from build123d import *

# Parameters (mm, degrees)
CROQUIS3_W                 = 106
CROQUIS3_H                 = 179
SALIENTE_EXTRUIR4_DEPTH    = 3
CROQUIS3_6_W               = 99.5
CROQUIS3_6_H               = 172.5
CROQUIS3_6_W_2             = 96.25
CROQUIS3_6_H_2             = 169.25
SALIENTE_EXTRUIR5_DEPTH    = 7
CROQUIS7_R                 = 10
CORTAR_EXTRUIR1_DEPTH      = 7
REDONDEO1_R                = 3
CORTAR_EXTRUIR2_DEPTH      = 20
CORTAR_EXTRUIR2_DEPTH_BACK = 20
CROQUIS8_R                 = 1.5
CROQUIS12_R                = 3
CORTAR_EXTRUIR3_DEPTH      = 2
CROQUIS13_R                = 2.5
SALIENTE_EXTRUIR7_DEPTH    = 1
CORTAR_EXTRUIR4_DEPTH      = 1
CORTAR_EXTRUIR4_DEPTH_BACK = 11
CROQUIS14_R                = 1.5


with BuildPart() as part:
    # Croquis3 → Saliente-Extruir4 (new body)
    with BuildSketch(Plane(origin=(0, 0, 0), x_dir=(1, 0, 0), z_dir=(0, 1, 0))):
        Rectangle(CROQUIS3_W, CROQUIS3_H)
    extrude(amount=SALIENTE_EXTRUIR4_DEPTH)

    # Croquis3_6 → Saliente-Extruir5 (add)
    with BuildSketch(Plane(origin=(0, 0, 0), x_dir=(1, 0, 0), z_dir=(0, 1, 0))):
        Rectangle(CROQUIS3_6_W, CROQUIS3_6_H)
        Rectangle(CROQUIS3_6_W_2, CROQUIS3_6_H_2, mode=Mode.SUBTRACT)
    extrude(amount=SALIENTE_EXTRUIR5_DEPTH)

    # Croquis7 → Cortar-Extruir1 (cut)
    with BuildSketch(Plane.XZ):
        with Locations(Location((28, -44.5, 0), (0, 0, 270))):
            Circle(CROQUIS7_R)
    extrude(amount=-CORTAR_EXTRUIR1_DEPTH, mode=Mode.SUBTRACT)

    # Redondeo1
    redondeo1_edges = [part.edges().sort_by_distance(p)[0] for p in [
        (53, 1.5, 89.5),
        (-53, 1.5, 89.5),
        (-53, 1.5, -89.5),
        (53, 1.5, -89.5),
    ]]
    fillet(redondeo1_edges, radius=REDONDEO1_R)

    # Croquis8 → Cortar-Extruir2 (cut, two sides: drawn at the far end of the back side and taken through both)
    with BuildSketch(Plane(origin=(0, 3, 0), x_dir=(1, 0, 0), z_dir=(0, 1, 0)).offset(-CORTAR_EXTRUIR2_DEPTH_BACK)):
        with Locations(Location((-34, 71, 0), (0, 0, 270))):
            Circle(CROQUIS8_R)
        with Locations(Location((34, 71, 0), (0, 0, 270))):
            Circle(CROQUIS8_R)
        with Locations(Location((-34, -70, 0), (0, 0, 270))):
            Circle(CROQUIS8_R)
        with Locations(Location((34, -70, 0), (0, 0, 270))):
            Circle(CROQUIS8_R)
    extrude(amount=CORTAR_EXTRUIR2_DEPTH + CORTAR_EXTRUIR2_DEPTH_BACK, mode=Mode.SUBTRACT)

    # Croquis12 → Cortar-Extruir3 (cut)
    with BuildSketch(Plane.XZ):
        with Locations(Location((-34, 70, 0), (0, 0, 270))):
            Circle(CROQUIS12_R)
        with Locations(Location((34, 70, 0), (0, 0, 270))):
            Circle(CROQUIS12_R)
        with Locations(Location((34, -71, 0), (0, 0, 270))):
            Circle(CROQUIS12_R)
        with Locations(Location((-34, -71, 0), (0, 0, 270))):
            Circle(CROQUIS12_R)
    extrude(amount=-CORTAR_EXTRUIR3_DEPTH, mode=Mode.SUBTRACT)

    # Croquis13 → Saliente-Extruir7 (add)
    with BuildSketch(Plane(origin=(0, 3, 0), x_dir=(1, 0, 0), z_dir=(0, 1, 0))):
        with Locations(Location((-34, 71, 0), (0, 0, 270))):
            Circle(CROQUIS13_R)
        with Locations(Location((34, 71, 0), (0, 0, 270))):
            Circle(CROQUIS13_R)
        with Locations(Location((-34, -70, 0), (0, 0, 270))):
            Circle(CROQUIS13_R)
        with Locations(Location((34, -70, 0), (0, 0, 270))):
            Circle(CROQUIS13_R)
    extrude(amount=SALIENTE_EXTRUIR7_DEPTH)

    # Croquis14 → Cortar-Extruir4 (cut, two sides: drawn at the far end of the back side and taken through both)
    with BuildSketch(Plane.XZ.offset(-CORTAR_EXTRUIR4_DEPTH_BACK)):
        with Locations(Location((-34, 70, 0), (0, 0, 270))):
            Circle(CROQUIS14_R)
        with Locations(Location((34, 70, 0), (0, 0, 270))):
            Circle(CROQUIS14_R)
        with Locations(Location((34, -71, 0), (0, 0, 270))):
            Circle(CROQUIS14_R)
        with Locations(Location((-34, -71, 0), (0, 0, 270))):
            Circle(CROQUIS14_R)
    extrude(amount=CORTAR_EXTRUIR4_DEPTH + CORTAR_EXTRUIR4_DEPTH_BACK, mode=Mode.SUBTRACT)


solid = part.part
Could you check a few things on this model? Use its own coordinates, in mm. A direction names the side the tool comes from. Give positions to 0.01 mm unless a question says otherwise; leave off trailing zeros. Order: outer loops, then holes, each group sorted by start corner. A loop starts at its lowest first (then second) coordinate and runs counter-clockwise, first axis right, second up. Notation, with made-up numbers: M -38.5,38 L 12.5,38 A12 cw 12.5,61 Z; hole C 89.5,39 d8. An arc over 180 degrees is marked long. One line per question, with ' | ' between items.
1. We'd pull the mould along X, two halves only. Please class faces 1 (the face through (-1, 0, -1)), 2 (the face through (-31.97, 0.99, 72.21)), 3 (the face through (-49.75, 5, 1)), 4 (the face through (35.69, 3.49, 68.16)): +X half, -X half, draft (parallel to the pull), parting line (faces both ways), or undercut.
Results:
face 1: draft | face 2: undercut | face 3: -X half | face 4: undercut
2. I want a section at C-C (z = -18.5). List the corners of the cut face in (x, y) for me (3 decimals).
Results:
outline: M -53,0 L 53,0 L 53,3 L 49.75,3 L 49.75,7 L 48.125,7 L 48.125,3 L -48.125,3 L -48.125,7 L -49.75,7 L -49.75,3 L -53,3 Z
3. I want a section at A-A (z = -44.5). List the corners of the cut face in (x, y) for me (3 decimals), and give its area (3 significant figures).
Results:
outline: M -53,0 L 18,0 L 18,3 L -48.125,3 L -48.125,7 L -49.75,7 L -49.75,3 L -53,3 Z; M 38,0 L 53,0 L 53,3 L 49.75,3 L 49.75,7 L 48.125,7 L 48.125,3 L 38,3 Z | area: 271 mm²
4. If I drill on line 1 (X direction, y = 0.5, z = 70); line 2 (Z direction, x = -37, y = 5) (3 decimals); line 3 (X direction, y = 4.5, z = 17.5) (3 decimals), over which ranges is the centre line in solid material (lowest first)?
Results:
line 1: -53 to -37, -31 to 31, 37 to 53 | line 2: -86.25 to -84.625, 84.625 to 86.25 | line 3: -49.75 to -48.125, 48.125 to 49.75
5. I want a section at B-B (x = -22). List the corners of the cut face in (y, z) for me (3 decimals), and give its area (3 significant figures).
Results:
outline: M 0,-89.5 L 3,-89.5 L 3,-86.25 L 7,-86.25 L 7,-84.625 L 3,-84.625 L 3,84.625 L 7,84.625 L 7,86.25 L 3,86.25 L 3,89.5 L 0,89.5 Z | area: 550 mm²
6. I'm going to push flat-ended pins straight in: pin 1 (1.2 mm diameter, centred on y = 5.5, z = -29.5, fed in from -X); pin 2 (1.2 mm diameter, centred on y = 4, z = -42.5, fed in from +X); pin 3 (5 mm diameter, centred on x = -11.5, z = 37.5, fed in from +Y); pin 4 (1.5 mm diameter, centred on x = 34, z = -71.5, fed in from +Y) (1 decimal). Where does each tip first touch, or does it pass through?
Results:
pin 1: x = -49.75 | pin 2: x = 49.75 | pin 3: y = 3 | pin 4: through
7. For faces 5 (the face through (-1, 5, 86.25)), 6 (the face through (32.7, 2, 68.7)), 7 (the face through (-34, 4, -69)), 8 (the face through (21.92, 1.48, -36.56)), which set-ups out of +Z, -Z, +X, -X, +Y, -Y let a thin tool reach every point of the face, with its end or its side?
Results:
face 5: +Z, +X, -X, +Y | face 6: -Y | face 7: +Y | face 8: +Y, -Y
